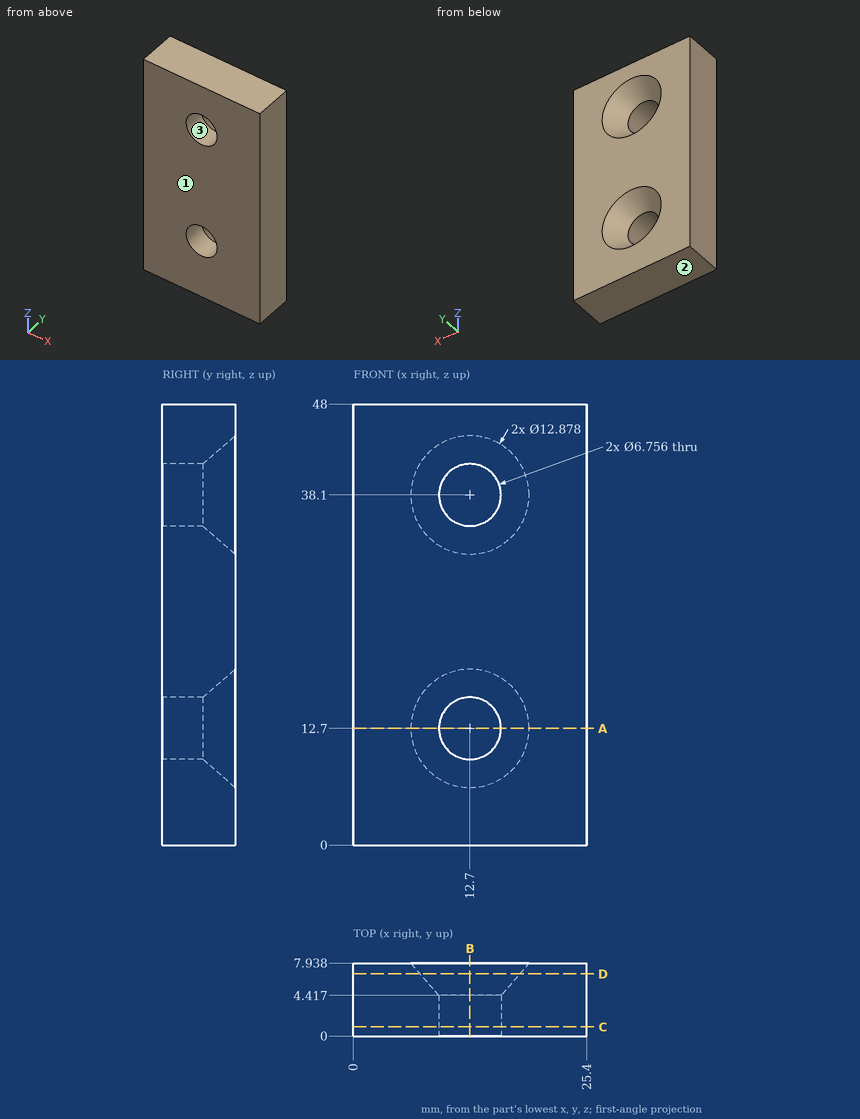
Study the drawing (mm; zero at the part's minimum x, y, z) and answer. Give positions to 0.01 mm unless a question says otherwise; leave off trailing zeros. Order: outer loops, then holes, each group sorted by start corner. A loop starts at its lowest first (then second) coordinate and runs counter-clockwise, first axis right, second up. Notation, with made-up numbers: M 42,-6.75 L 54,-6.75 A27 ccw 54,10.25 Z; hole C -6,-16 d8. An arc over 180 degrees is marked long. Put each result on its own line as item: value. Start each with the question number.
Item 1: Find the intervals of material crossed by line 1 along Z through (x, y) = (12.7, 2.6); line 2 along X through (y, z) = (1.25, 38.1); line 3 along Z through (x, y) = (11, 5.5), in increasing order.
Item 2: The part is cut by section A-A, the plane z = 12.7. Determine the outline of the cut face in (x, y), and give its area (3 significant figures).
Item 3: The part is cut by section D-D, the plane y = 6.75. Determine the outline of the cut face in (x, z).
Item 4: For a pull along Z with two mould halves and no side action, classify the marked faces 1, 2 and 3 as +Z half, -Z half, draft (parallel to the pull), parting line (faces both ways), or undercut.
Item 5: The part is cut by section C-C, the plane y = 1. Determine the outline of the cut face in (x, z).
Item 6: The part is cut by section B-B, the plane x = 12.7. Determine the outline of the cut face in (y, z).
Answer key:
1. line 1: z = 0 to 9.32, 16.08 to 34.72, 41.48 to 48
1. line 2: x = 0 to 9.32, 16.08 to 25.4
1. line 3: z = 0 to 8.73, 16.67 to 34.13, 42.07 to 48
2. outline: M 0,0 L 9.32,0 L 9.32,4.42 L 6.26,7.94 L 0,7.94 Z; M 16.08,0 L 25.4,0 L 25.4,7.94 L 19.14,7.94 L 16.08,4.42 Z
2. area: 137 mm²
3. outline: M 0,0 L 25.4,0 L 25.4,48 L 0,48 Z; hole C 12.7,12.7 d10.81; hole C 12.7,38.1 d10.81
4. face 1: draft
4. face 2: -Z half
4. face 3: undercut
5. outline: M 0,0 L 25.4,0 L 25.4,48 L 0,48 Z; hole C 12.7,12.7 d6.76; hole C 12.7,38.1 d6.76
6. outline: M 0,0 L 7.94,0 L 7.94,6.26 L 4.42,9.32 L 0,9.32 Z; M 0,16.08 L 4.42,16.08 L 7.94,19.14 L 7.94,31.66 L 4.42,34.72 L 0,34.72 Z; M 0,41.48 L 4.42,41.48 L 7.94,44.54 L 7.94,48 L 0,48 Z
